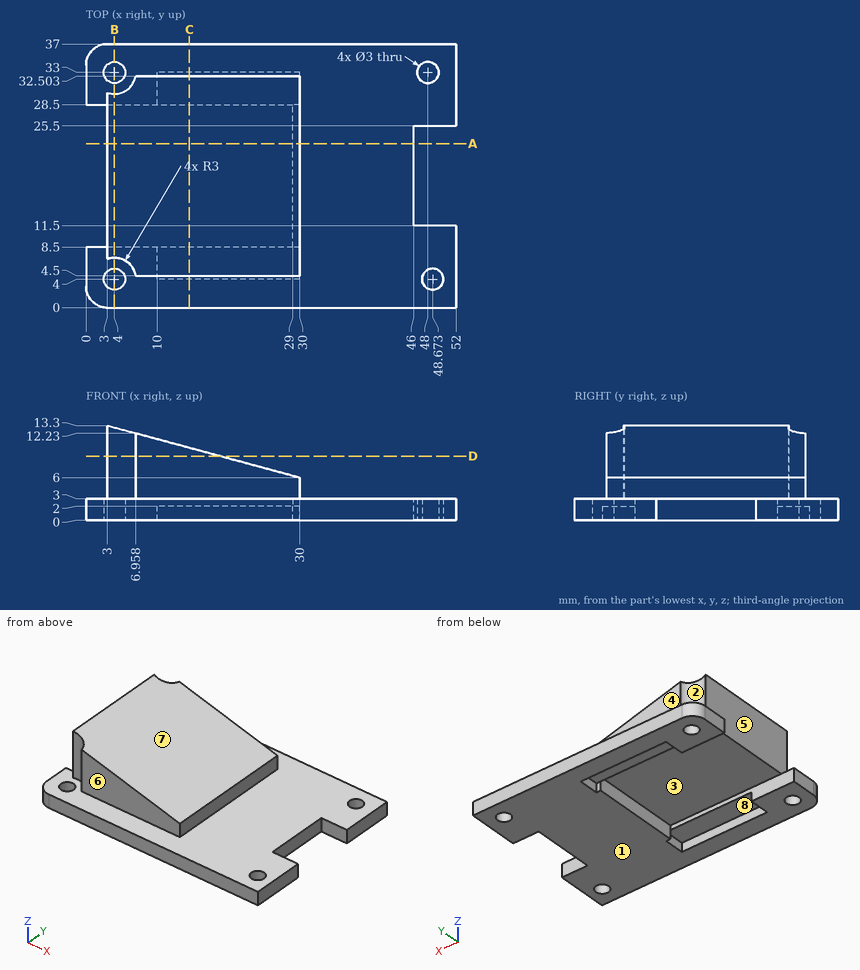
Geometry check sheet. Reference: drawing and pictorial views, mm from the part's lowest x, y, z. A direction names the side the tool comes from. Coordinates: 2 decimals unless noted, no trailing zeros. Write each loop counter-clockwise with the first axis right and the second up, starting at its lowest first coordinate (ties: lowest second). Pieces come first, ordered by that corner, then holes. Notation, with made-up numbers: (51.5, -35) -> (87.5, -35) arc R25 cw to (87.5, -21) -> close; hole circle Ø1 at (2.25, 18.5). An arc over 180 degrees is marked (long way). Use a Markdown table: item, result.
1. Sectioned sample at D-D (z = 9). Enter the section's corners in (x, y) (1 decimal).
Reported:
| item | result |
|---|---|
| outline | (3, 6.8) arc R3 cw to (7, 4.5) -> (18.9, 4.5) -> (18.9, 32.5) -> (7, 32.5) arc R3 cw to (3, 30.2) -> close |
2. Tool access check on the marked faces 1, 2, 3 and 4. Record the directions out of +Z, -Z, +X, -X, +Y, -Y that give a thin tool (end or side, any length) a straight path to the whole face; none if there is none.
Reported:
| item | result |
|---|---|
| face 1 | -Z, +X, -X, +Y, -Y |
| face 2 | +Z, +Y |
| face 3 | -Z, -X |
| face 4 | +Z, +X, -X, +Y |
3. Go/stop test with flat-tipped pins: pin 1 Ø1.5 at (y, z) = (24, 4) entering from +X; pin 2 Ø6 at (x, y) = (26.5, 24.5) entering from +Z; pin 3 Ø1.5 at (x, y) = (8.5, 21.5) entering from +Z (1 decimal). Record where each tip stops, or that it passes through.
Reported:
| item | result |
|---|---|
| pin 1 | stops at x = 30 |
| pin 2 | stops at z = 7.76 |
| pin 3 | stops at z = 12 |
4. Release check for a two-part mould opening along X. For the marked faces 5, 6, 7 and 8 record: pulls with the +X half, pulls with the -X half, needs draft (parallel to the pull), parting line crosses it, or undercut.
Reported:
| item | result |
|---|---|
| face 5 | pulls with the -X half |
| face 6 | needs draft |
| face 7 | pulls with the +X half |
| face 8 | undercut |
5. Sectioned sample at A-A (y = 23). Enter the section's corners in (x, z).
Reported:
| item | result |
|---|---|
| outline | (3, 3) -> (29, 3) -> (29, 0) -> (46, 0) -> (46, 3) -> (30, 3) -> (30, 6) -> (3, 13.3) -> close |
6. Sectioned sample at B-B (x = 4). Enter the section's corners in (y, z).
Reported:
| item | result |
|---|---|
| outline | (0, 0) -> (2.5, 0) -> (2.5, 3) -> (0, 3) -> close; (5.5, 0) -> (8.5, 0) -> (8.5, 3) -> (28.5, 3) -> (28.5, 0) -> (31.5, 0) -> (31.5, 3) -> (30, 3) -> (30, 13.03) -> (7, 13.03) -> (7, 3) -> (5.5, 3) -> close; (34.5, 0) -> (37, 0) -> (37, 3) -> (34.5, 3) -> close |
7. Sectioned sample at C-C (x = 14.5). Enter the section's corners in (y, z).
Reported:
| item | result |
|---|---|
| outline | (0, 0) -> (4, 0) -> (4, 2) -> (8.5, 2) -> (8.5, 3) -> (28.5, 3) -> (28.5, 2) -> (33, 2) -> (33, 0) -> (37, 0) -> (37, 3) -> (32.5, 3) -> (32.5, 10.19) -> (4.5, 10.19) -> (4.5, 3) -> (0, 3) -> close |
8. Scan lines: line 1 along X through (y, z) = (33, 2.1); line 2 along Y through (x, z) = (4, 1.3); line 3 along Y through (x, z) = (49, 2) (1 decimal). Record each from-to range of solid material in increasing order.
Reported:
| item | result |
|---|---|
| line 1 | x = 0 to 2.5, 5.5 to 46.5, 49.5 to 52 |
| line 2 | y = 0 to 2.5, 5.5 to 8.5, 28.5 to 31.5, 34.5 to 37 |
| line 3 | y = 0 to 2.5, 5.5 to 11.5, 25.5 to 31.9, 34.1 to 37 |
